Solid Edge part; units mm, degrees
sketch "Sketch1" plane through (0, 0, 0) normal (0, 0, 1) x (1, 0, 0)
  line L0 (-12.4629, 15.7402) -> (-2.138, -1.2958)
  arc A0 (-2.138, -1.2958) -> (2.498, -0.1) centre (0, 0) ccw
  arc A1 (4.9286, 13.1207) -> (2.498, -0.1) centre (50.0083, -2.001) ccw
  line L1 (3.7627, 14.3543) -> (0.8885, 3.3896)
  arc A2 (-1.3853, 3.2186) -> (0.8885, 3.3896) centre (-0.2778, 3.6953) ccw
  line L2 (-7.8069, 18.1385) -> (-1.3853, 3.2186)
  arc A3 (3.7627, 14.3543) -> (4.9286, 13.1207) centre (4.73, 14.1008) cw
  arc A4 (-12.4629, 15.7402) -> (-7.8068, 18.1385) centre (-10.218, 17.1008) cw
extrude "Protrusion1" add sketch "Sketch1" along normal blind 8
hole "Agujero_1" at (0, 0, 8) direction (0, 0, -1) diameter 3.2 end up to next
sketch "Sketch2" plane through (-3.5565, 8.6129, 8) normal (0, 0, 1) x (-0.2535623, -0.9673191, 0)
  line L0 (0.7294, -4.8844) -> (-2.0582, -1.782)
  line L1 (-8.1366, -6.5268) -> (-2.0582, -1.782)
  arc A0 (-4.6361, -10.4226) -> (-8.1366, -6.5268) centre (-6.5214, -8.596) cw
  line L2 (-4.6361, -10.4226) -> (0.7294, -4.8844)
extrude "VaciadoExtruido_3" cut sketch "Sketch2" against normal blind 6
chamfer "Chaflán_5" distance 0.5 angle 45 8 edges at (-7.3004, 7.2222, 0) (0.6244, -2.4208, 0) (3.2438, 6.5967, 0) (-11.4201, 19.4344, 0) (-4.5961, 10.6786, 0) (-0.1874, 2.493, 0) (2.3256, 8.8719, 0) (5.4568, 14.7876, 0)
sketch "Sketch3" plane through (0, 0, 4) normal (0, 0, 1) x (1, 0, 0)
  circle A0 centre (-10.218, 17.1008) radius 1.5
extrude "Cutout1" cut sketch "Sketch3" against normal through all
sketch "Sketch4" plane through (2.3256, 8.8719, 4.75) normal (-0.9673191, 0.2535623, 0) x (-0.2535623, -0.9673191, 0)
  line L0 (5.6676, 3.25) -> (-6.6676, -2.75)
extrude "Cutout2" cut sketch "Sketch4" against normal through all material side at (2.4579, 9.3767, 5.045)
sketch "Sketch5" plane through (-4.5961, 10.6786, 4.25) normal (0.9185349, 0.3953399, 0) x (-0.3953399, 0.9185349, 0)
  line L0 (0.4106, 3.75) -> (0.4106, -2.25)
  line L1 (-8.1216, 3.75) -> (0.4106, -2.25)
  line L2 (-8.1216, 3.75) -> (0.4106, 3.75)
sketch "Sketch6" plane through (-7.3004, 7.2222, 4.25) normal (-0.8551957, -0.5183052, 0) x (0.5183052, -0.8551957, 0)
  line L0 (6.4897, 3.75) -> (-2.2493, 3.75)
  line L1 (-2.2493, 3.75) -> (-2.2493, -2.25)
  line L2 (-2.2493, -2.25) -> (6.4897, 3.75)
loft "LoftedCutout1" cut profiles "Sketch5", "Sketch6"
fillet "Redondeo_6" radius 4 2 edges at (-2.6611, 2.4454, 8) (1.8014, 3.1503, 8)
Verification items for the finished model (mm, model axes). A direction names the side the tool comes from. Give positions to 0.01 mm unless a question says otherwise; leave off trailing zeros. Order: outer loops, then holes, each group sorted by start corner. A loop starts at its lowest first (then second) coordinate and runs counter-clockwise, first axis right, second up. Notation, with made-up numbers: M -18.75,42 L 20.25,42 A20 ccw 20.25,61 Z; hole C -4.5,16.5 d3. An arc over 180 degrees is marked long. Answer as a JSON object with one key per item and string values. Group by question number.
1) Depth check by flat-ended pin: pin 1 Ø1.5 at (x, z) = (-4.5, 1) entering from -Y; pin 2 Ø3.5 at (x, y) = (-10.22, 17.1) entering from +Z; pin 3 Ø4 at (x, z) = (-5, 6.5) entering from -Y. Enter the tip coordinate at first touch or a pass-through.
2) Mould release check, pull along Y, two halves, no side actions. Record for faces 4 (the face through (-0.167, 2.495, 4.198)), 5 (the face through (-9, 15, 2)), 6 (the face through (-8.83, 16.53, 1.01)): released by +Y, released by -Y, zero draft, split by the parting line, or undercut.
3) Scan lines: line 1 along Z through (x, y) = (-9, 13.5); line 2 along X through (y, z) = (0.75, 7.25); line 3 along X through (y, z) = (10.25, 1.5). Record each from-to range of solid material in increasing order. Write a range as [from, to].
4) Access from +Z, -Z, +X, -X, +Y, -Y to the whole of each face (thin tool, end or side, straight path). Record for faces 1 (the face through (2.551, 8.731, 0.246)), 2 (the face through (-3.93, 9.13, 2.47)), 3 (the face through (0.7, -2.4, 4.2)).
5) Cross-section at A-A (z = 1.5). Enter the section's corners in (x, y) (3 decimals).
Result sheet:
{
 "1": {"pin 1": "stops at y = 1.36", "pin 2": "stops at z = 2", "pin 3": "stops at y = 0.13"},
 "2": {"face 4": "released by +Y", "face 5": "zero draft", "face 6": "undercut"},
 "3": {"line 1": "z = [0, 2]", "line 2": "x = [-3.38, -1.41], [1.41, 2.54]", "line 3": "x = [-9.14, -4.41], [2.69, 4.07]"},
 "4": {"face 1": "-Z, +Y", "face 2": "+Z, -Z, +Y", "face 3": "+Z, -Z, -Y"},
 "5": {"outline": "M -12.463,15.74 L -2.138,-1.296 A2.5 ccw 2.498,-0.1 A47.548 cw 4.929,13.121 A1 ccw long 3.763,14.354 L 0.889,3.39 A1.206 cw -1.385,3.219 L -7.807,18.139 A2.625 ccw long Z; hole C -10.218,17.101 d3; hole C 0,0 d3.2"}
}
